Design review of the part built by this model. Coordinates are the model's own, in mm. A direction names the side the tool comes from. Give positions to 0.01 mm unless a question says otherwise; leave off trailing zeros. Write each loop counter-clockwise with the first axis right and the second up, starting at its lowest first coordinate (ties: lowest second). Pieces come first, ordered by that corner, then holes. Notation, with made-up numbers: M 78,64 L 129,64 A12 cw 129,87 Z; hole C -13,-1 d5. An arc over 180 degrees is marked long. Answer in a Markdown table with one row per item.
```python
from build123d import *

# Parameters (mm, degrees)
EXTRUDE_1_DEPTH     = 5
EXTRUDE_3_DEPTH     = 30
SKETCH_6_R          = 4
SKETCH_6_R_2        = 2
EXTRUDE_4_DEPTH     = 10
CUT_EXTRUDE_1_DEPTH = 10
CUT_EXTRUDE_3_DEPTH = 10
CUT_EXTRUDE_4_DEPTH = 15


with BuildPart() as part:
    # 草图1 → 凸台-拉伸1 (new body)
    with BuildSketch(Plane(origin=(0, 0, 0), x_dir=(1, 0, 0), z_dir=(0, 1, 0))):
        Polygon((45, 18.639610307), (18.639610307, 45), (-18.639610307, 45), (-45, 18.639610307), (-45, -18.639610307), (-18.639610307, -45), (18.639610307, -45), (45, -18.639610307), align=None)
    extrude(amount=EXTRUDE_1_DEPTH)

    # 草图5 → 凸台-拉伸3 (add)
    with BuildSketch(Plane(origin=(0, 5, 0), x_dir=(1, 0, 0), z_dir=(0, 1, 0))):
        Polygon((45, -18.639610307), (45, 18.639610307), (18.639610307, 45), (-18.639610307, 45), (-45, 18.639610307), (-45, -18.639610307), (-18.639610307, -45), (18.639610307, -45), align=None)
        Polygon((41, 16.982756057), (16.982756057, 41), (-16.982756057, 41), (-41, 16.982756057), (-41, -16.982756057), (-16.982756057, -41), (16.982756057, -41), (41, -16.982756057), align=None, mode=Mode.SUBTRACT)
    extrude(amount=EXTRUDE_3_DEPTH)

    # 草图6 → 凸台-拉伸4 (add)
    # profile 1 of 3: a face of its own
    with BuildSketch(Plane(origin=(0, 5, 0), x_dir=(1, 0, 0), z_dir=(0, 1, 0))):
        with Locations(Location((-17, 33, 0), (0, 0, 270))):
            Circle(SKETCH_6_R)
        with Locations(Location((-17, 33, 0), (0, 0, 270))):
            Circle(SKETCH_6_R_2, mode=Mode.SUBTRACT)
    # profile 2 of 3: a face of its own
    with BuildSketch(Plane(origin=(0, 5, 0), x_dir=(1, 0, 0), z_dir=(0, 1, 0))):
        with Locations(Location((10, -33, 0), (0, 0, 270))):
            Circle(SKETCH_6_R)
        with Locations(Location((10, -33, 0), (0, 0, 270))):
            Circle(SKETCH_6_R_2, mode=Mode.SUBTRACT)
    # profile 3 of 3: a face of its own
    with BuildSketch(Plane(origin=(0, 5, 0), x_dir=(1, 0, 0), z_dir=(0, 1, 0))):
        with Locations(Location((-22, -22, 0), (0, 0, 270))):
            Circle(SKETCH_6_R)
        with Locations(Location((-22, -22, 0), (0, 0, 270))):
            Circle(SKETCH_6_R_2, mode=Mode.SUBTRACT)
    extrude(amount=EXTRUDE_4_DEPTH)

    # 草图7 → 切除-拉伸1 (cut)
    with BuildSketch(Plane(origin=(0, 5, 0), x_dir=(1, 0, 0), z_dir=(0, 1, 0))):
        with BuildLine():
            ThreePointArc((10.5, 3), (11.914213562, 2.414213562), (12.5, 1))
            Line((12.5, 1), (12.5, -1))
            ThreePointArc((12.5, -1), (11.914213562, -2.414213562), (10.5, -3))
            Line((10.5, -3), (-10.5, -3))
            ThreePointArc((-10.5, -3), (-11.914213562, -2.414213562), (-12.5, -1))
            Line((-12.5, -1), (-12.5, 1))
            ThreePointArc((-12.5, 1), (-11.914213562, 2.414213562), (-10.5, 3))
            Line((-10.5, 3), (10.5, 3))
        make_face()
    extrude(amount=-CUT_EXTRUDE_1_DEPTH, mode=Mode.SUBTRACT)

    # 草图10 → 切除-拉伸3 (cut)
    with BuildSketch(Plane.ZY.offset(45)):
        with BuildLine():
            Line((0, 20), (14, 20))
            ThreePointArc((14, 20), (14.707106781, 20.292893219), (15, 21))
            Line((15, 21), (15, 24))
            ThreePointArc((15, 24), (14.707106781, 24.707106781), (14, 25))
            Line((14, 25), (-14, 25))
            ThreePointArc((-14, 25), (-14.707106781, 24.707106781), (-15, 24))
            Line((-15, 24), (-15, 21))
            ThreePointArc((-15, 21), (-14.707106781, 20.292893219), (-14, 20))
            Line((-14, 20), (0, 20))
        make_face()
    extrude(amount=-CUT_EXTRUDE_3_DEPTH, mode=Mode.SUBTRACT)

    # 草图11 → 切除-拉伸4 (cut)
    with BuildSketch(Plane(origin=(0, 35, 0), x_dir=(1, 0, 0), z_dir=(0, 1, 0))):
        Polygon((41, 0), (41, 10), (45, 10), (45, -10), (41, -10), align=None)
    extrude(amount=-CUT_EXTRUDE_4_DEPTH, mode=Mode.SUBTRACT)


solid = part.part
```
1) For faces 4 (the face through (-22, 5, 22)), 5 (the face through (-11.93, 2.54, -2.4)), 6 (the face through (43, 20, 0)), list the 3-axis set-ups (+Z, -Z, +X, -X, +Y, -Y) from which the entire face can be reached by the end or side of a thin tool; tool diameter is ignored.
Geometry says:
| item | result |
|---|---|
| face 4 | +Y |
| face 5 | +Y, -Y |
| face 6 | +X, -X, +Y |
2) Add section D-D (x = 31). Write out the cut boundary in (y, z), and give its area (3 significant figures).
Geometry says:
| item | result |
|---|---|
| outline | M 0,-32.64 L 35,-32.64 L 35,-26.98 L 5,-26.98 L 5,26.98 L 35,26.98 L 35,32.64 L 0,32.64 Z |
| area | 666 mm^2 |
3) Add section B-B (x = -6.5). Write out the cut boundary in (y, z), and give its area (3 significant figures).
Geometry says:
| item | result |
|---|---|
| outline | M 0,-45 L 35,-45 L 35,-41 L 5,-41 L 5,-3 L 0,-3 Z; M 0,3 L 5,3 L 5,41 L 35,41 L 35,45 L 0,45 Z |
| area | 660 mm^2 |
4) Insertion check: P1, Ø2.5, axis at x = -43, y = 23, coming from the -Z side; P2, Ø6.5, axis at x = 8, z = 35, coming from the +Y side; P3, Ø2, axis at x = -29.5, y = 6, coming from the -Z side. Each pin has a flat end and moves straight along its axis. Give the tip position at first contact, or say it passes through.
Geometry says:
| item | result |
|---|---|
| P1 | z = -21.89 |
| P2 | y = 15 |
| P3 | z = -35.14 |
5) Add section A-A (y = 13). Write out the cut boundary in (x, z).
Geometry says:
| item | result |
|---|---|
| outline | M -45,-18.64 L -18.64,-45 L 18.64,-45 L 45,-18.64 L 45,18.64 L 18.64,45 L -18.64,45 L -45,18.64 Z; C -22,22 d8; C -17,-33 d8; C 10,33 d8; hole M -41,-16.98 L -16.98,-41 L 16.98,-41 L 41,-16.98 L 41,16.98 L 16.98,41 L -16.98,41 L -41,16.98 Z; hole C -22,22 d4; hole C -17,-33 d4; hole C 10,33 d4 |
6) To check wall thickness, follow probe 1 along Z at (x, y) = (-8.5, 29.5); probe 2 along X at (y, z) = (9, 22). State the ranges of each line that lie inside material, in increasing order. Write a range as [from, to].
Geometry says:
| item | result |
|---|---|
| probe 1 | [-45, -41], [41, 45] |
| probe 2 | [-41.64, -35.98], [-26, -24], [-20, -18], [35.98, 41.64] |
7) The part is to be moulded in two halves that separate along Y. For faces 1 (the face through (-43, 23, -15)), 2 (the face through (-1, 5, -10)), 3 (the face through (0, 3, 3)), say which applies: released by +Y, released by -Y, zero draft, split by the parting line, or undercut.
Geometry says:
| item | result |
|---|---|
| face 1 | undercut |
| face 2 | released by +Y |
| face 3 | zero draft |
8) Add section C-C (z = -33). Write out the cut boundary in (x, y).
Geometry says:
| item | result |
|---|---|
| outline | M -30.64,0 L 30.64,0 L 30.64,35 L 24.98,35 L 24.98,5 L -13,5 L -13,15 L -15,15 L -15,5 L -19,5 L -19,15 L -21,15 L -21,5 L -24.98,5 L -24.98,35 L -30.64,35 Z |
